from build123d import *

# Parameters (mm, degrees)
SCHIZZO1_W                   = 252
SCHIZZO1_H                   = 400
ESTRUSIONE_ESTRUSIONE1_DEPTH = 20
SCHIZZO3_W                   = 60
SCHIZZO3_H                   = 12.0854414
TAGLIO_ESTRUSIONE1_DEPTH     = 420.852355001
SCHIZZO4_R                   = 3.3
TAGLIO_ESTRUSIONE2_DEPTH     = 238.027951938
SCHIZZO5_R                   = 3
TAGLIO_ESTRUSIONE3_DEPTH     = 238.225630993
SCHIZZO6_R                   = 3
SCHIZZO6_R_2                 = 2.5
TAGLIO_ESTRUSIONE4_DEPTH     = 238.225630993


with BuildPart() as part:
    # Schizzo1 → Estrusione-Estrusione1 (new body)
    with BuildSketch(Plane.XY):
        Rectangle(SCHIZZO1_W, SCHIZZO1_H)
    extrude(amount=ESTRUSIONE_ESTRUSIONE1_DEPTH)

    # Schizzo3 → Taglio-Estrusione1 (cut, through all)
    with BuildSketch(Plane(origin=(0, 200, 0), x_dir=(1, 0, 0), z_dir=(0, 1, 0))):
        with Locations((0, -23.5427207)):
            Rectangle(SCHIZZO3_W, SCHIZZO3_H)
    extrude(amount=-TAGLIO_ESTRUSIONE1_DEPTH, mode=Mode.SUBTRACT)

    # Schizzo4 → Taglio-Estrusione2 (cut, through all)
    with BuildSketch(Plane.XY.offset(17.5)):
        with Locations((22.92355164, 190)):
            Circle(SCHIZZO4_R)
        with Locations((-23.07644836, 190)):
            Circle(SCHIZZO4_R)
        with Locations((22.92355164, -155)):
            Circle(SCHIZZO4_R)
        with Locations((-23.07644836, -155)):
            Circle(SCHIZZO4_R)
        with Locations((22.92355164, -168)):
            Circle(SCHIZZO4_R)
        with Locations((-23.07644836, -168)):
            Circle(SCHIZZO4_R)
    extrude(amount=-TAGLIO_ESTRUSIONE2_DEPTH, mode=Mode.SUBTRACT)

    # Schizzo5 → Taglio-Estrusione3 (cut, through all)
    with BuildSketch(Plane.XY.offset(20)):
        with Locations((80.500605801, -120)):
            Circle(SCHIZZO5_R)
        with Locations((80.500605801, -180)):
            Circle(SCHIZZO5_R)
        with Locations((80.500605801, 180)):
            Circle(SCHIZZO5_R)
        with Locations((80.500605801, 120)):
            Circle(SCHIZZO5_R)
        with Locations((80.500605801, 60)):
            Circle(SCHIZZO5_R)
        with Locations((80.500605801, 0)):
            Circle(SCHIZZO5_R)
        with Locations((80.500605801, -60)):
            Circle(SCHIZZO5_R)
    taglio_estrusione3 = extrude(amount=-TAGLIO_ESTRUSIONE3_DEPTH, mode=Mode.SUBTRACT)

    # Specchia1: Taglio-Estrusione3 across plane
    add(taglio_estrusione3.mirror(Plane(origin=(0, 0, 0), x_dir=(0, 0, 1), z_dir=(1, 0, 0))), mode=Mode.SUBTRACT)

    # Schizzo6 → Taglio-Estrusione4 (cut, through all)
    with BuildSketch(Plane.XY.offset(20)):
        with Locations((108, 92.808299679)):
            Circle(SCHIZZO6_R)
        with Locations((63, 92.808299679)):
            Circle(SCHIZZO6_R)
        with Locations((108, 149.808299679)):
            Circle(SCHIZZO6_R)
        with Locations((63, 149.808299679)):
            Circle(SCHIZZO6_R)
        with Locations((-3.5, 95.308299679)):
            Circle(SCHIZZO6_R_2)
        with Locations((18.5, 95.308299679)):
            Circle(SCHIZZO6_R_2)
        with Locations((-3.5, 57.308299679)):
            Circle(SCHIZZO6_R_2)
        with Locations((18.5, 57.308299679)):
            Circle(SCHIZZO6_R_2)
        with Locations((-63, 92.808299679)):
            Circle(SCHIZZO6_R)
        with Locations((-108, 92.808299679)):
            Circle(SCHIZZO6_R)
        with Locations((-63, 149.808299679)):
            Circle(SCHIZZO6_R)
        with Locations((-108, 149.808299679)):
            Circle(SCHIZZO6_R)
    extrude(amount=-TAGLIO_ESTRUSIONE4_DEPTH, mode=Mode.SUBTRACT)


solid = part.part
Work out the finished part from the listing and answer in its coordinate system (mm). Round coordinates to 2 decimals unless told otherwise and drop trailing zeros. Loops run counter-clockwise (first coordinate to the right, second up) from the corner with the lowest first, then second, coordinate; pieces in that order, holes last. Notation, with made-up numbers: (-29, 12) - (-24, 12) arc R18 cw to (-24, 38) - close; hole circle Ø6 at (51.25, 34.25). An arc over 180 degrees is marked (long way). One line per item, written item: value.
Q1. Each of these flat-tipped pins is pushed along its axis until it touches: pin 1 Ø5.5 at (x, y) = (-63, 149.81) entering from -Z; pin 2 Ø4 at (x, y) = (-60.5, -86) entering from -Z; pin 3 Ø10.5 at (x, y) = (22.92, -155) entering from +Z. Where does it stop, or does it pass through?
Check values:
pin 1: through
pin 2: z = 0
pin 3: z = 17.5
Q2. Straight lines are drawn through the part: probe 1 along X at (y, z) = (180, 10); probe 2 along Y at (x, z) = (108.5, 15.5); probe 3 along X at (y, z) = (-20, 19.25). For each, find the intervals that lie inside material, in ascending order.
Check values:
probe 1: -126 to -83.5, -77.5 to 77.5, 83.5 to 126
probe 2: -200 to 89.85, 95.77 to 146.85, 152.77 to 200
probe 3: -126 to -30, 30 to 126
Q3. Find section A-A on y = -69.5. Give the vertices of the cut face in (x, z), and give its area (3 significant figures).
Check values:
outline: (-126, 0) - (126, 0) - (126, 20) - (30, 20) - (30, 17.5) - (-30, 17.5) - (-30, 20) - (-126, 20) - close
area: 4,890 mm2
Q4. The mould has two halves that part along X. Classify faces 1 (the flat face through (-2, 3, 0)), 2 (the flat face through (-126, -3, 10)), 3 (the flat face through (0, 3, 17.5)): +X half, -X half, draft (parallel to the pull), parting line (faces both ways), or undercut.
Check values:
face 1: draft
face 2: -X half
face 3: undercut
